For this review, take the finished solid that the model builds, in its own axes (mm). Coordinates: 2 decimals unless noted, no trailing zeros. Loops run counter-clockwise (first coordinate to the right, second up) from the corner with the lowest first, then second, coordinate; pieces in that order, holes last.
```python
from build123d import *

# Parameters (mm, degrees)
SKETCH_1_W               = 80
SKETCH_1_H               = 80
EXTRUDE_1_DEPTH          = 2.5
SKETCH_2_R               = 1.5
CUT_EXTRUDE_1_DEPTH      = 10
PATTERN_CIRCULAR_1_COUNT = 4


with BuildPart() as part:
    # Эскиз1 → Бобышка-Вытянуть1 (new body)
    with BuildSketch(Plane(origin=(0, 0, 0), x_dir=(1, 0, 0), z_dir=(0, 1, 0))):
        Rectangle(SKETCH_1_W, SKETCH_1_H)
    extrude(amount=EXTRUDE_1_DEPTH)

    # Эскиз2 → Вырез-Вытянуть1 (cut)
    with BuildSketch(Plane(origin=(0, 2.5, 0), x_dir=(1, 0, 0), z_dir=(0, 1, 0))):
        with Locations(Location((-15, -37, 0), (0, 0, 270))):
            Circle(SKETCH_2_R)
        with Locations(Location((15, -37, 0), (0, 0, 270))):
            Circle(SKETCH_2_R)
    cut_extrude_1 = extrude(amount=-CUT_EXTRUDE_1_DEPTH, mode=Mode.SUBTRACT)

    # Круговой массив1: Вырез-Вытянуть1 ×4 about axis
    pattern_circular_1_axis = Axis((0, 0, -0.081911433), (0, 1, 0))
    for i in range(1, PATTERN_CIRCULAR_1_COUNT):
        add(cut_extrude_1.rotate(pattern_circular_1_axis, i * 360 / PATTERN_CIRCULAR_1_COUNT), mode=Mode.SUBTRACT)


solid = part.part
```
Q1. The part is to be moulded in two halves that separate along X. For faces 1 (the face through (-1, 1, -40)), 2 (the face through (-15.9, 1.3, 35.8)), 3 (the face through (37.77, 1.27, -13.75)), 4 (the face through (-40, 1, 1)), say which applies: +X half, -X half, draft (parallel to the pull), parting line (faces both ways), or undercut.
Q2. For pin 1 Ø1.8 at (x, z) = (-15, -37.16) entering from +Y; pin 2 Ø5 at (x, z) = (-37.08, -15.08) entering from +Y, all flat-tipped, find the tip position at first contact; note any pin that passes through.
Q3. Consider section B-B (x = 15). State the section outline as (y, z) points.
Q4. Wall thickness on probe 1 along X at (y, z) = (0.9, 37); probe 2 along X at (y, z) = (2.35, 16): over which ranges is each line inside the solid? List them lowest first.
Q5. Consider section A-A (z = 37). State the section outline as (x, y) points.
Model answer:
1. face 1: draft
1. face 2: undercut
1. face 3: undercut
1. face 4: -X half
2. pin 1: passes through
2. pin 2: stops at y = 2.5
3. outline: (0, -40) - (2.5, -40) - (2.5, -38.66) - (0, -38.66) - close; (0, -35.66) - (2.5, -35.66) - (2.5, 35.5) - (0, 35.5) - close; (0, 38.5) - (2.5, 38.5) - (2.5, 40) - (0, 40) - close
4. probe 1: x = -40 to -16.5, -13.5 to 13.5, 16.5 to 40
4. probe 2: x = -40 to -38.12, -36.04 to 36.04, 38.12 to 40
5. outline: (-40, 0) - (-16.5, 0) - (-16.5, 2.5) - (-40, 2.5) - close; (-13.5, 0) - (13.5, 0) - (13.5, 2.5) - (-13.5, 2.5) - close; (16.5, 0) - (40, 0) - (40, 2.5) - (16.5, 2.5) - close
